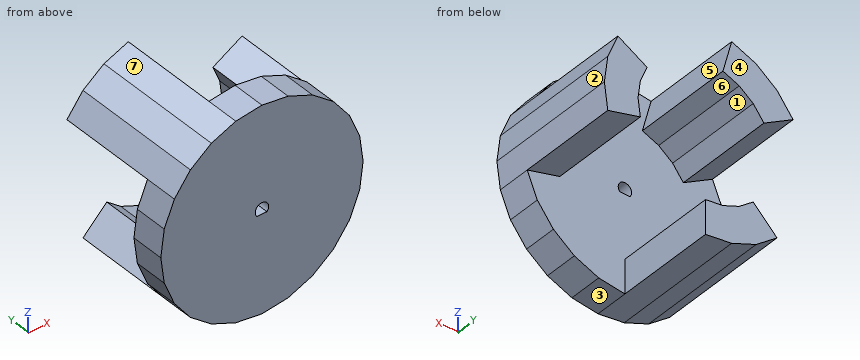
```python
from build123d import *

# Parameters (mm, degrees)
BOSS_EXTRUDE2_DEPTH = 10
BOSS_EXTRUDE3_DEPTH = 40
BOSS_EXTRUDE4_DEPTH = 10


with BuildPart() as part:
    # Sketch1 → Boss-Extrude2 (new body)
    with BuildSketch(Plane(origin=(0, 0, 0), x_dir=(1, 0, 0), z_dir=(0, 1, 0))):
        Polygon((-10.087889227, 17.472736683), (-14.266429761, 14.266429761), (-17.472736683, 10.087889227), (-19.488305475, 5.221875714), (-20.175778455, 0), (-19.488305475, -5.221875714), (-17.472736683, -10.087889227), (-14.266429761, -14.266429761), (-10.087889227, -17.472736683), (-5.221875714, -19.488305475), (0, -20.175778455), (5.221875714, -19.488305475), (10.087889227, -17.472736683), (14.266429761, -14.266429761), (17.472736683, -10.087889227), (19.488305475, -5.221875714), (20.175778455, 0), (19.488305475, 5.221875714), (17.472736683, 10.087889227), (14.266429761, 14.266429761), (10.087889227, 17.472736683), (5.221875714, 19.488305475), (0, 20.175778455), (-5.221875714, 19.488305475), align=None)
        with BuildLine():
            Line((-1.497847768, 1.325312063), (1.497847768, 1.325312063))
            ThreePointArc((1.497847768, 1.325312063), (0, -2), (-1.497847768, 1.325312063))
        make_face(mode=Mode.SUBTRACT)
    extrude(amount=BOSS_EXTRUDE2_DEPTH)

    # Sketch1_5 → Boss-Extrude3 (add)
    with BuildSketch(Plane(origin=(0, 0, 0), x_dir=(1, 0, 0), z_dir=(0, 1, 0))):
        Polygon((-17.472736683, -10.087889227), (-14.266429761, -14.266429761), (-10.087889227, -17.472736683), (-5.221875714, -19.488305475), (-7.82919648, -29.218959046), (-15.124846159, -26.197002003), (-21.389762566, -21.389762566), (-26.197002003, -15.124846159), align=None)
        Polygon((0, 20.175778455), (-5.221875714, 19.488305475), (-10.087889227, 17.472736683), (-14.266429761, 14.266429761), (-21.389762566, 21.389762566), (-15.124846159, 26.197002003), (-7.82919648, 29.218959046), (0, 30.249692317), align=None)
        Polygon((17.472736683, -10.087889227), (19.488305475, -5.221875714), (20.175778455, 0), (19.488305475, 5.221875714), (29.218959046, 7.82919648), (30.249692317, 0), (29.218959046, -7.82919648), (26.197002003, -15.124846159), align=None)
    extrude(amount=BOSS_EXTRUDE3_DEPTH)

    # Sketch1_7 → Boss-Extrude4 (add)
    with BuildSketch(Plane(origin=(0, 0, 0), x_dir=(1, 0, 0), z_dir=(0, 1, 0))):
        Polygon((-17.472736683, -10.087889227), (-26.197002003, -15.124846159), (-29.218959046, -7.82919648), (-30.249692317, 0), (-29.218959046, 7.82919648), (-26.197002003, 15.124846159), (-21.389762566, 21.389762566), (-14.266429761, 14.266429761), (-17.472736683, 10.087889227), (-19.488305475, 5.221875714), (-20.175778455, 0), (-19.488305475, -5.221875714), align=None)
        Polygon((19.488305475, 5.221875714), (17.472736683, 10.087889227), (14.266429761, 14.266429761), (10.087889227, 17.472736683), (5.221875714, 19.488305475), (0, 20.175778455), (0, 30.249692317), (7.82919648, 29.218959046), (15.124846159, 26.197002003), (21.389762566, 21.389762566), (26.197002003, 15.124846159), (29.218959046, 7.82919648), align=None)
        Polygon((-5.221875714, -19.488305475), (0, -20.175778455), (5.221875714, -19.488305475), (10.087889227, -17.472736683), (14.266429761, -14.266429761), (17.472736683, -10.087889227), (26.197002003, -15.124846159), (21.389762566, -21.389762566), (15.124846159, -26.197002003), (7.82919648, -29.218959046), (0, -30.249692317), (-7.82919648, -29.218959046), align=None)
    extrude(amount=BOSS_EXTRUDE4_DEPTH)


solid = part.part
```
The model under review builds one solid part; all positions refer to its coordinate system, in mm. Face numbers are marked on the shaded views. A direction names the side the tool comes from. Round coordinates to 2 decimals unless told otherwise and drop trailing zeros. Order: outer loops, then holes, each group sorted by start corner. A loop starts at its lowest first (then second) coordinate and runs counter-clockwise, first axis right, second up.
Item 1: Draft analysis for pull direction Z (two halves, no side actions). For the marked faces 1, 2, 3 and 4, state which applies: released by +Z, released by -Z, zero draft, split by the parting line, or undercut.
Working result:
face 1: undercut
face 2: released by +Z
face 3: released by -Z
face 4: zero draft
Item 2: Add section B-B, the plane y = 9. State the section outline as (x, z) points, and give its area (3 significant figures).
Working result:
outline: (-30.25, 0) - (-29.22, -7.83) - (-26.2, -15.12) - (-21.39, -21.39) - (-15.12, -26.2) - (-7.83, -29.22) - (0, -30.25) - (7.83, -29.22) - (15.12, -26.2) - (21.39, -21.39) - (26.2, -15.12) - (29.22, -7.83) - (30.25, 0) - (29.22, 7.83) - (26.2, 15.12) - (21.39, 21.39) - (15.12, 26.2) - (7.83, 29.22) - (0, 30.25) - (-7.83, 29.22) - (-15.12, 26.2) - (-21.39, 21.39) - (-26.2, 15.12) - (-29.22, 7.83) - close; hole (-1.5, -1.33) - (1.5, -1.33) arc R2 ccw (long way) to start
area: 2,830 mm2
Item 3: To check wall thickness, follow probe 1 along X at (y, z) = (6, 0); probe 2 along Y at (x, z) = (-18, -11.5); probe 3 along Z at (x, y) = (-21, 16). State the ranges of each line that lie inside material, in increasing order.
Working result:
probe 1: x = -30.25 to -2, 2 to 30.25
probe 2: y = 0 to 10
probe 3: z = -21.69 to -21, 12.12 to 21.69
Item 4: For pin 1 (1 mm diameter, centred on x = -3.5, y = 4.5, fed in from -Z); pin 2 (8 mm diameter, centred on y = 27.5, z = -27.5, fed in from +X); pin 3 (4 mm diameter, centred on y = 11.5, z = 22.5, fed in from -X), all flat-tipped, find the tip position at first contact; note any pin that passes through.
Working result:
pin 1: stops at z = -29.85
pin 2: stops at x = 0
pin 3: stops at x = -22.07
Item 5: Add section C-C, the plane z = -3.5. State the section outline as (x, y) points (3 decimals), and give its area (3 significant figures).
Working result:
outline: (-29.789, 0) - (29.789, 0) - (29.789, 40) - (19.715, 40) - (19.715, 10) - (-29.789, 10) - close
area: 898 mm2
Item 6: Add section D-D, the plane z = 11.5. State the section outline as (x, y) points.
Working result:
outline: (-27.7, 0) - (27.7, 0) - (27.7, 40) - (19.92, 40) - (19.92, 10) - (-16.39, 10) - (-16.39, 40) - (-19.92, 40) - (-19.92, 10) - (-27.7, 10) - close
Item 7: Add section A-A, the plane y = 13.5. State the section outline as (x, z) points, and give its area (3 significant figures).
Working result:
outline: (-26.2, 15.12) - (-17.47, 10.09) - (-14.27, 14.27) - (-10.09, 17.47) - (-5.22, 19.49) - (-7.83, 29.22) - (-15.12, 26.2) - (-21.39, 21.39) - close; (-21.39, -21.39) - (-15.12, -26.2) - (-7.83, -29.22) - (0, -30.25) - (0, -20.18) - (-5.22, -19.49) - (-10.09, -17.47) - (-14.27, -14.27) - close; (17.47, 10.09) - (19.49, 5.22) - (20.18, 0) - (19.49, -5.22) - (29.22, -7.83) - (30.25, 0) - (29.22, 7.83) - (26.2, 15.12) - close
area: 592 mm2
Item 8: Machinability: for the marked faces 5, 6 and 7, which of the approach directions +Z, -Z, +X, -X, +Y, -Y give a long, thin tool a straight path to every point of the face, cutting with its end or side? Answer none if there is none.
Working result:
face 5: +Z, +X, +Y
face 6: +X, +Y
face 7: +Z, -X, +Y, -Y
